Source: three-view drawing plus pictorial views. Frame: mm from the lowest corner of the part. A direction names the side the tool comes from. Coordinates: 2 decimals unless noted, no trailing zeros. Order: outer loops, then holes, each group sorted by start corner. A loop starts at its lowest first (then second) coordinate and runs counter-clockwise, first axis right, second up. Notation, with made-up numbers: (44.25, -31) - (51.25, -31) arc R15 cw to (51.25, -23) - close; hole circle Ø4 at (69.25, -33.75). An arc over 180 degrees is marked (long way). One line per question, with ' | ' between items.
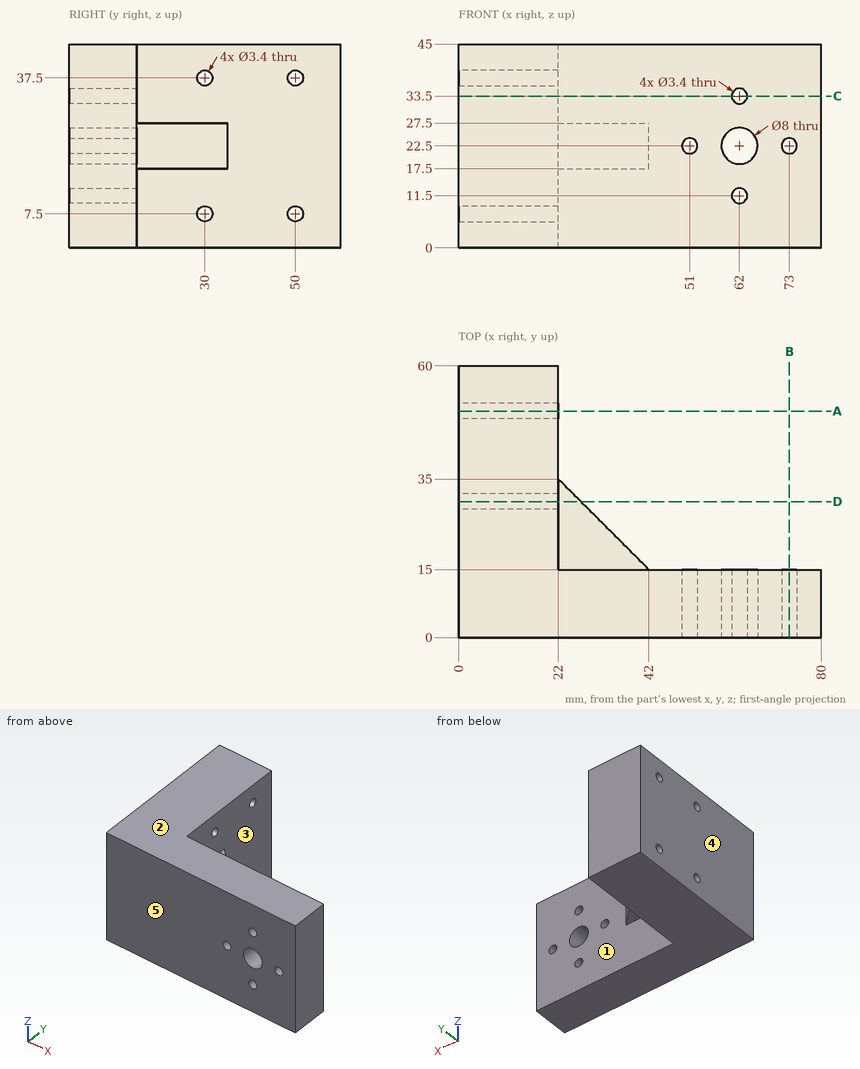
Item 1: Section B-B on x = 73. Return the cut outline in (y, z).
Data:
outline: (0, 0) - (15, 0) - (15, 20.8) - (0, 20.8) - close; (0, 24.2) - (15, 24.2) - (15, 45) - (0, 45) - close
Item 2: Section A-A on y = 50. Return the cut outline in (x, z), and give its area (3 significant figures).
Data:
outline: (0, 0) - (22, 0) - (22, 5.8) - (0, 5.8) - close; (0, 9.2) - (22, 9.2) - (22, 35.8) - (0, 35.8) - close; (0, 39.2) - (22, 39.2) - (22, 45) - (0, 45) - close | area: 840 mm^2
Item 3: Draft query along X for the marked faces 3, 4 and 5. Return one class per face: released by +X, released by -X, zero draft, split by the parting line, or undercut.
Data:
face 3: released by +X | face 4: released by -X | face 5: zero draft
Item 4: Ray query, line 1 (Z direction, x = 62, y = 7.5); line 2 (X direction, y = 8.5, z = 22.5); line 3 (Z direction, x = 13, y = 30). Return the intervals inside material, ascending.
Data:
line 1: 0 to 9.8, 13.2 to 18.5, 26.5 to 31.8, 35.2 to 45 | line 2: 0 to 49.3, 52.7 to 58, 66 to 71.3, 74.7 to 80 | line 3: 0 to 5.8, 9.2 to 35.8, 39.2 to 45
Item 5: Section D-D on y = 30. Return the cut outline in (x, z), and give its area (3 significant figures).
Data:
outline: (0, 0) - (22, 0) - (22, 5.8) - (0, 5.8) - close; (0, 9.2) - (22, 9.2) - (22, 17.5) - (27, 17.5) - (27, 27.5) - (22, 27.5) - (22, 35.8) - (0, 35.8) - close; (0, 39.2) - (22, 39.2) - (22, 45) - (0, 45) - close | area: 890 mm^2
Item 6: Access query for the marked faces 1 and 2. Directions: +Z, -Z, +X, -X, +Y, -Y. A direction counts if a zero-diameter tool reaches every point of the face in a straight line with its end or side. Return the directions, or none.
Data:
face 1: +X, +Y | face 2: +Z, +X, -X, +Y, -Y
Item 7: Contact query for flat-ended pins moving along their axis: P1, Ø2, axis at y = 50, z = 37.5, coming from the +X side; P2, Ø22.5, axis at x = 40, z = 29.5, coming from the +Y side; P3, Ø10, axis at y = 52.5, z = 8.5, coming from the +X side; P4, Ø13, axis at x = 62, z = 22.5, coming from the +Y side. Output: stop coordinate, or through.
Data:
P1: through | P2: y = 28.07 | P3: x = 22 | P4: y = 15
Item 8: Section C-C on z = 33.5. Return the cut outline in (x, y), and give its area (3 significant figures).
Data:
outline: (0, 0) - (60.3, 0) - (60.3, 15) - (22, 15) - (22, 60) - (0, 60) - close; (63.7, 0) - (80, 0) - (80, 15) - (63.7, 15) - close | area: 2,140 mm^2
